Verification items for the finished model (mm, model axes). A direction names the side the tool comes from. Give positions to 0.01 mm unless a question says otherwise; leave off trailing zeros. Loops run counter-clockwise (first coordinate to the right, second up) from the corner with the lowest first, then second, coordinate; pieces in that order, holes last. Notation, with made-up numbers: M 2.5,18.5 L 15.5,18.5 A23 cw 15.5,56.5 Z; hole C 88.5,-24.5 d9. An arc over 180 degrees is marked long. Answer in a Markdown table with one row per item.
```python
from build123d import *

# Parameters (mm, degrees)
SKETCH1_W                 = 14.859
SKETCH1_H                 = 107.315
BOSS_EXTRUDE1_DEPTH       = 9.398
SKETCH2_W                 = 6.35
SKETCH2_H                 = 13.335
CUT_EXTRUDE1_DEPTH        = 109.242376411
F_5_CLEARANCE_HOLE1_D     = 3.556
F_5_CLEARANCE_HOLE1_DEPTH = 1.524
F_5_CLEARANCE_HOLE2_D     = 3.556
F_5_CLEARANCE_HOLE2_DEPTH = 14.859
F_5_CLEARANCE_HOLE3_D     = 3.556
F_5_CLEARANCE_HOLE3_DEPTH = 9.398
FILLET1_R                 = 0.635


with BuildPart() as part:
    # Sketch1 → Boss-Extrude1 (new body)
    with BuildSketch(Plane(origin=(4.699, 0, 0), x_dir=(0, 0, -1), z_dir=(1, 0, 0))):
        with Locations((5.9055, 53.6575)):
            Rectangle(SKETCH1_W, SKETCH1_H)
    extrude(amount=-BOSS_EXTRUDE1_DEPTH)

    # Sketch2 → Cut-Extrude1 (cut, through all)
    with BuildSketch(Plane.XZ):
        with Locations((0, -6.6675)):
            Rectangle(SKETCH2_W, SKETCH2_H)
    extrude(amount=-CUT_EXTRUDE1_DEPTH, mode=Mode.SUBTRACT)

    # #5 Clearance Hole1
    with Locations(Plane(origin=(-3.175, 0, 0), x_dir=(0, 0, -1), z_dir=(1, 0, 0))):
        with Locations((8.5725, 92.7735), (8.5725, 102.5525), (8.5725, 82.9945), (8.5725, 73.2155), (8.5725, 63.4365), (8.5725, 53.6575), (8.5725, 43.8785), (8.5725, 34.0995), (8.5725, 24.3205), (8.5725, 14.5415), (8.5725, 4.7625)):
            Hole(F_5_CLEARANCE_HOLE1_D / 2, depth=F_5_CLEARANCE_HOLE1_DEPTH)

    # #5 Clearance Hole2
    with Locations(Plane.XY.offset(1.524)):
        with Locations((0, 92.7735), (0, 102.5525), (0, 82.9945), (0, 73.2155), (0, 63.4365), (0, 53.6575), (0, 43.8785), (0, 34.0995), (0, 24.3205), (0, 14.5415), (0, 4.7625)):
            Hole(F_5_CLEARANCE_HOLE2_D / 2, depth=F_5_CLEARANCE_HOLE2_DEPTH)

    # #5 Clearance Hole3
    with Locations(Plane(origin=(4.699, 0, 0), x_dir=(0, 0, -1), z_dir=(1, 0, 0))):
        with Locations((8.5725, 92.7735), (8.5725, 102.5525), (8.5725, 82.9945), (8.5725, 73.2155), (8.5725, 63.4365), (8.5725, 53.6575), (8.5725, 43.8785), (8.5725, 34.0995), (8.5725, 24.3205), (8.5725, 14.5415), (8.5725, 4.7625)):
            Hole(F_5_CLEARANCE_HOLE3_D / 2, depth=F_5_CLEARANCE_HOLE3_DEPTH)

    # Fillet1
    fillet1_edges = [part.edges().sort_by_distance(p)[0] for p in [
        (3.937, 0, -13.335),
        (3.937, 107.315, -13.335),
        (-3.937, 107.315, -13.335),
        (-3.937, 0, -13.335),
    ]]
    fillet(fillet1_edges, radius=FILLET1_R)


solid = part.part
```
Item 1: Scan lines: L1, parallel to X at y = 69, z = -5 (3 decimals); L2, parallel to X at y = 93, z = 0.75; L3, parallel to Z at x = -3, y = 80.5. Record each from-to range of solid material in increasing order. Write a range as [from, to].
Reported:
| item | result |
|---|---|
| L1 | x = [-4.699, -3.175], [3.175, 4.699] |
| L2 | x = [-4.7, -1.76], [1.76, 4.7] |
| L3 | z = [0, 1.52] |
Item 2: Release check for a two-part mould opening along Z. For faces 3 (the flat face through (4.699, 54, -6)), 4 (the cylindrical face through (-3.948, 51.922, -8.958)), 5 (the flat face through (2, 53, 0)) record: released by +Z, released by -Z, zero draft, split by the parting line, or undercut.
Reported:
| item | result |
|---|---|
| face 3 | zero draft |
| face 4 | undercut |
| face 5 | released by -Z |
Item 3: Go/stop test with flat-tipped pins: pin 1 (5.5 mm diameter, centred on y = 53.66, z = -8.57, fed in from +X); pin 2 (5.5 mm diameter, centred on x = 0, y = 34.1, fed in from -Z). Record where each tip stops, or that it passes through.
Reported:
| item | result |
|---|---|
| pin 1 | stops at x = 4.7 |
| pin 2 | stops at z = 0 |
Item 4: Sectioned sample at A-A (z = -3). Record the cut outline in (x, y) (3 decimals).
Reported:
| item | result |
|---|---|
| outline | M -4.699,0 L -3.175,0 L -3.175,107.315 L -4.699,107.315 Z; M 3.175,0 L 4.699,0 L 4.699,107.315 L 3.175,107.315 Z |
Item 5: Sectioned sample at B-B (y = 90). Record the cut outline in (x, z) (3 decimals), and give its area (3 significant figures).
Reported:
| item | result |
|---|---|
| outline | M -4.699,-13.335 L -3.175,-13.335 L -3.175,0 L 3.175,0 L 3.175,-13.335 L 4.699,-13.335 L 4.699,1.524 L -4.699,1.524 Z |
| area | 55.0 mm^2 |
Item 6: Tool access check on faces 1 (the cylindrical face through (3.926, 22.743, -7.752)), 2 (the flat face through (-3.175, 52.91, -6.76)). Record the directions out of +Z, -Z, +X, -X, +Y, -Y that give a thin tool (end or side, any length) a straight path to the whole face; none if there is none.
Reported:
| item | result |
|---|---|
| face 1 | +X, -X |
| face 2 | -Z, +Y, -Y |
Item 7: Sectioned sample at C-C (x = 0). State how many separate pieces and enclosed holes the cut face has, and give its area (3 significant figures).
Reported:
| item | result |
|---|---|
| separate pieces | 12 |
| enclosed holes | 0 |
| area | 104 mm^2 |
